CAD build for the part. Positions are in the model's coordinates, mm. A direction names the side the tool comes from. Coordinates: 2 decimals unless noted, no trailing zeros. Loops run counter-clockwise (first coordinate to the right, second up) from the corner with the lowest first, then second, coordinate; pieces in that order, holes last. Notation, with made-up numbers: (7, -5) -> (22, -5) arc R26 ccw to (22, 20) -> close; hole circle Ø10 at (66.25, 18.5). An arc over 180 degrees is marked (long way). Answer as a JSON object with one key per item and string values. Group by question number.
from build123d import *

# Parameters (mm, degrees)
F0_W     = 210
F0_H     = 2.6
F1_DEPTH = 1.5
F0_H_2   = 4.2
F2_DEPTH = 8
F3_R     = 4


with BuildPart() as f1:
    # F0 (on Top) → F1 (new body)
    with BuildSketch(Plane.XY):
        Rectangle(F0_W, F0_H)
    extrude(amount=F1_DEPTH)

    # F0 (on Top) → F2 (join)
    with BuildSketch(Plane.XY):
        with Locations((0, 3.4)):
            Rectangle(F0_W, F0_H_2)
        with Locations((0, -3.4)):
            Rectangle(F0_W, F0_H_2)
    extrude(amount=F2_DEPTH)

    # F3
    f3_edges = [f1.edges().sort_by_distance(p)[0] for p in [
        (0, 5.5, 8),
        (0, -5.5, 8),
    ]]
    fillet(f3_edges, radius=F3_R)


solid = f1.part
Item 1: Flat gauge pin, fed straight in: P1, Ø1.3, axis at x = 21.5, y = 0.5, coming from the +Z side. Where does the tip first touch, or does it go through?
Item 2: Pull direction Y, two halves, no side cores. Call faces 3 (the flat face through (-1, 1.3, 5)), 4 (the cylindrical face through (1.47, -4.297, 6.859)), 5 (the cylindrical face through (1.47, 4.359, 6.797)): +Y half, -Y half, draft (parallel to the pull), parting line (faces both ways), or undercut.
Item 3: 3-axis set-ups, long thin cutter, end or side, ignore diameter. For faces 1 (the flat face through (-1, -5.5, 2)), 2 (the flat face through (-1, -1.3, 5)): which of +Z, -Z, +X, -X, +Y, -Y reach the whole face in a straight line?
Item 4: Band-saw the part on A-A, the plane z = 2.75. List the corners of the cut face in (x, y).
Item 5: Drill centre lines: L1, parallel to Y at x = 42, z = 3; L2, parallel to Z at x = 66.5, y = -0.25; L3, parallel to Y at x = 30.5, z = 5.75. Where is each one in solid material? Low to high.
Item 6: Band-saw the part on B-B, the plane x = 47.5. List the corners of the cut face in (y, z), and give its area (3 significant figures).
Item 7: Band-saw the part on C-C, the plane y = -3.25. List the corners of the cut face in (x, z).
Reply:
{
 "1": {"P1": "z = 1.5"},
 "2": {"face 3": "undercut", "face 4": "-Y half", "face 5": "+Y half"},
 "3": {"face 1": "+Z, -Z, +X, -X, -Y", "face 2": "+Z, +X, -X"},
 "4": {"outline": "(-105, -5.5) -> (105, -5.5) -> (105, -1.3) -> (-105, -1.3) -> close; (-105, 1.3) -> (105, 1.3) -> (105, 5.5) -> (-105, 5.5) -> close"},
 "5": {"L1": "-5.5 to -1.3, 1.3 to 5.5", "L2": "0 to 1.5", "L3": "-5.1 to -1.3, 1.3 to 5.1"},
 "6": {"outline": "(-5.5, 0) -> (5.5, 0) -> (5.5, 4) arc R4 ccw to (1.5, 8) -> (1.3, 8) -> (1.3, 1.5) -> (-1.3, 1.5) -> (-1.3, 8) -> (-1.5, 8) arc R4 ccw to (-5.5, 4) -> close", "area": "64.2 mm²"},
 "7": {"outline": "(-105, 0) -> (105, 0) -> (105, 7.6) -> (-105, 7.6) -> close"}
}
